CAD build for the part. Positions are in the model's coordinates, mm. A direction names the side the tool comes from. Round coordinates to 2 decimals unless told otherwise and drop trailing zeros. Loops run counter-clockwise (first coordinate to the right, second up) from the corner with the lowest first, then second, coordinate; pieces in that order, holes last.
```python
from build123d import *

# Parameters (mm, degrees)
SKETCH1_W           = 25
SKETCH1_H           = 38
BOSS_EXTRUDE1_DEPTH = 40
SKETCH2_R           = 3
CUT_EXTRUDE1_DEPTH  = 39
SKETCH4_R           = 4.15
CUT_EXTRUDE2_DEPTH  = 41
CUT_EXTRUDE3_DEPTH  = 18
SKETCH6_R           = 1.6
CUT_EXTRUDE4_DEPTH  = 41
SKETCH7_W           = 18
SKETCH7_H           = 32
CUT_EXTRUDE5_DEPTH  = 3
SKETCH9_R           = 6
CUT_EXTRUDE6_DEPTH  = 1.5
SKETCH10_R          = 6
CUT_EXTRUDE7_DEPTH  = 1.5


with BuildPart() as part:
    # Sketch1 → Boss-Extrude1 (new body)
    with BuildSketch(Plane(origin=(0, 0, 0), x_dir=(1, 0, 0), z_dir=(0, 1, 0))):
        Rectangle(SKETCH1_W, SKETCH1_H)
    extrude(amount=BOSS_EXTRUDE1_DEPTH)

    # Sketch2 → Cut-Extrude1 (cut, through all)
    with BuildSketch(Plane.XY.offset(19)):
        with Locations((0, 32)):
            Circle(SKETCH2_R)
    extrude(amount=-CUT_EXTRUDE1_DEPTH, mode=Mode.SUBTRACT)

    # Sketch4 → Cut-Extrude2 (cut, through all)
    with BuildSketch(Plane(origin=(0, 40, 0), x_dir=(1, 0, 0), z_dir=(0, 1, 0))):
        with Locations((0, -8)):
            Circle(SKETCH4_R)
        with Locations((0, 8)):
            Circle(SKETCH4_R)
    extrude(amount=-CUT_EXTRUDE2_DEPTH, mode=Mode.SUBTRACT)

    # Sketch5 → Cut-Extrude3 (cut)
    with BuildSketch(Plane(origin=(0, 40, 0), x_dir=(1, 0, 0), z_dir=(0, 1, 0))):
        Polygon((-3.7, -14.408587988), (3.7, -14.408587988), (7.4, -8), (3.7, -1.591412012), (-3.7, -1.591412012), (-7.4, -8), align=None)
        Polygon((-3.7, 14.408587988), (-7.4, 8), (-3.7, 1.591412012), (3.7, 1.591412012), (7.4, 8), (3.7, 14.408587988), align=None)
    extrude(amount=-CUT_EXTRUDE3_DEPTH, mode=Mode.SUBTRACT)

    # Sketch6 → Cut-Extrude4 (cut, through all)
    with BuildSketch(Plane(origin=(0, 40, 0), x_dir=(1, 0, 0), z_dir=(0, 1, 0))):
        with Locations((9, -16)):
            Circle(SKETCH6_R)
        with Locations((-9, -16)):
            Circle(SKETCH6_R)
        with Locations((-9, 16)):
            Circle(SKETCH6_R)
        with Locations((9, 16)):
            Circle(SKETCH6_R)
    extrude(amount=-CUT_EXTRUDE4_DEPTH, mode=Mode.SUBTRACT)

    # Sketch7 → Cut-Extrude5 (cut)
    with BuildSketch(Plane(origin=(0, 40, 0), x_dir=(1, 0, 0), z_dir=(0, 1, 0))):
        Rectangle(SKETCH7_W, SKETCH7_H)
    extrude(amount=-CUT_EXTRUDE5_DEPTH, mode=Mode.SUBTRACT)

    # Sketch9 → Cut-Extrude6 (cut)
    with BuildSketch(Plane(origin=(0, 0, -19), x_dir=(-1, 0, 0), z_dir=(0, 0, -1))):
        with Locations((0, 32)):
            Circle(SKETCH9_R)
    extrude(amount=-CUT_EXTRUDE6_DEPTH, mode=Mode.SUBTRACT)

    # Sketch10 → Cut-Extrude7 (cut)
    with BuildSketch(Plane.XY.offset(19)):
        with Locations((0, 32)):
            Circle(SKETCH10_R)
    extrude(amount=-CUT_EXTRUDE7_DEPTH, mode=Mode.SUBTRACT)


solid = part.part
```
Item 1: Cut at A-A, the plane y = 20.5. Give the cut face in (x, z).
Answers follow:
outline: (-12.5, -19) - (12.5, -19) - (12.5, 19) - (-12.5, 19) - close; hole circle Ø3.2 at (-9, -16); hole circle Ø3.2 at (-9, 16); hole circle Ø8.3 at (0, -8); hole circle Ø8.3 at (0, 8); hole circle Ø3.2 at (9, -16); hole circle Ø3.2 at (9, 16)
Item 2: Cut at C-C, the plane z = -0.5. Give the cut face in (x, y), plus the area to 3 significant figures.
Answers follow:
outline: (-12.5, 0) - (12.5, 0) - (12.5, 40) - (9, 40) - (9, 37) - (-9, 37) - (-9, 40) - (-12.5, 40) - close; hole circle Ø6 at (0, 32)
area: 918 mm2
Item 3: Cut at D-D, the plane y = 37.5. Give the cut face in (x, z).
Answers follow:
outline: (-12.5, -19) - (-2.4, -19) - (-2.4, -17.5) - (2.4, -17.5) - (2.4, -19) - (12.5, -19) - (12.5, 19) - (2.4, 19) - (2.4, 17.5) - (-2.4, 17.5) - (-2.4, 19) - (-12.5, 19) - close; hole (-9, -14.4) arc R1.6 ccw (long way) to (-7.4, -16) - (7.4, -16) arc R1.6 ccw (long way) to (9, -14.4) - (9, 14.4) arc R1.6 ccw (long way) to (7.4, 16) - (-7.4, 16) arc R1.6 ccw (long way) to (-9, 14.4) - close
Item 4: 3-axis set-ups, long thin cutter, end or side, ignore diameter. For faces 5 (the flat face through (3, 31, -17.5)), 6 (the flat face through (0, 28, 14.409)), 7 (the cylindrical face through (-2.21, 34.03, 0.02)): which of +Z, -Z, +X, -X, +Y, -Y reach the whole face in a straight line?
Answers follow:
face 5: -Z
face 6: +Y
face 7: +Z, -Z
Item 5: Probe line 1 (X direction, y = 17, z = -16); line 2 (Z direction, x = 0, y = 10); line 3 (X direction, y = 37, z = -16.5). List the from-to ranges inside material, lowest first.
Answers follow:
line 1: x = -12.5 to -10.6, -7.4 to 7.4, 10.6 to 12.5
line 2: z = -19 to -12.15, -3.85 to 3.85, 12.15 to 19
line 3: x = -12.5 to -10.52, -7.48 to 7.48, 10.52 to 12.5
Item 6: Cut at B-B, the plane z = -5. Give the cut face in (x, y), plus the area to 3 significant figures.
Answers follow:
outline: (-12.5, 0) - (-2.87, 0) - (-2.87, 22) - (-5.67, 22) - (-5.67, 37) - (-9, 37) - (-9, 40) - (-12.5, 40) - close; (2.87, 0) - (12.5, 0) - (12.5, 40) - (9, 40) - (9, 37) - (5.67, 37) - (5.67, 22) - (2.87, 22) - close
area: 650 mm2
Item 7: Two-plate mould, pull along Y, no slides. Class faces 1 (the flat face through (0, 28, 1.591)), 2 (the cylindrical face through (-2.21, 34.03, -15.93)), 3 (the flat face through (3.2, 22, 5.1)), 4 (the flat face through (0, 0, 0)): released by +Y, released by -Y, zero draft, split by the parting line, or undercut.
Answers follow:
face 1: zero draft
face 2: undercut
face 3: released by +Y
face 4: released by -Y
Item 8: Flat gauge pins, fed straight in: P1, Ø10.5, axis at x = -1, z = -7.5, coming from the +Y side; P2, Ø3, axis at x = 2.5, y = 31.5, coming from the +Z side; P3, Ø11, axis at x = 0, y = 32, coming from the -Z side. Where does each tip first touch, or does it go through?
Answers follow:
P1: stops at y = 22
P2: stops at z = 17.5
P3: stops at z = -17.5
